Build history of the part. All positions in model axes, mm. Face numbers are marked on the shaded views. A direction names the side the tool comes from. Coordinates: 2 decimals unless noted, no trailing zeros.
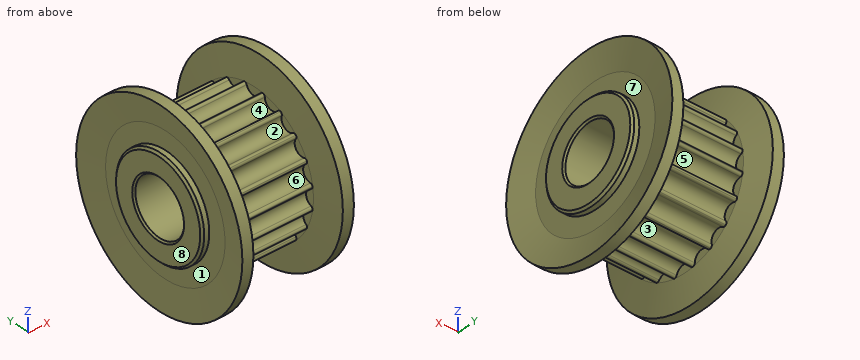
```python
from build123d import *

# Parameters (mm, degrees)
CUT_EXTRUDE_START        = 1.65
CUT_EXTRUDE_1_DEPTH      = 7
PATTERN_CIRCULAR_1_COUNT = 20
SKETCH_6_R               = 2.5
CUT_EXTRUDE_2_DEPTH      = 11.3
CHAMFER_1_SIZE           = 0.15


with BuildPart() as part:
    # Sketch 3 → Revolve 1 (revolve)
    with BuildSketch(Plane.XY):
        Polygon((0, 0), (0, 4.31), (0.19, 4.5), (1.65, 4.5), (1.65, 6.11), (8.65, 6.11), (8.65, 4.5), (10.11, 4.5), (10.3, 4.31), (10.3, 0), align=None)
    revolve(axis=Axis((10.3, 0, 0), (-1, 0, 0)))

    # Sketch 4 → Cut-Extrude 1 (cut)
    with BuildSketch(Plane(origin=(0, 0, 0), x_dir=(0, 0, -1), z_dir=(1, 0, 0)).offset(CUT_EXTRUDE_START)):
        with BuildLine():
            ThreePointArc((0.968009552, 6.032831633), (0.81174441, 6.002056879), (0.712936658, 5.877145279))
            ThreePointArc((0.712936658, 5.877145279), (0, 5.36), (-0.712936658, 5.877145279))
            ThreePointArc((-0.712936658, 5.877145279), (-0.81174441, 6.002056879), (-0.968009552, 6.032831633))
            ThreePointArc((-0.968009552, 6.032831633), (0, 6.11), (0.968009552, 6.032831633))
        make_face()
    cut_extrude_1 = extrude(amount=CUT_EXTRUDE_1_DEPTH, mode=Mode.SUBTRACT)

    # Pattern Circular 1: Cut-Extrude 1 ×20 about axis
    pattern_circular_1_axis = Axis((0, 0, 0), (1, 0, 0))
    for i in range(1, PATTERN_CIRCULAR_1_COUNT):
        add(cut_extrude_1.rotate(pattern_circular_1_axis, i * 360 / PATTERN_CIRCULAR_1_COUNT), mode=Mode.SUBTRACT)

    # Sketch 5 → Revolve 2 (revolve)
    with BuildSketch(Plane.XY):
        Polygon((1.1, 8.5), (1.65, 6.11), (1.65, 4.5), (0.65, 4.5), (0.65, 6.11), (0.1, 8.5), align=None)
        Polygon((9.65, 4.5), (8.65, 4.5), (8.65, 6.11), (9.2, 8.5), (10.2, 8.5), (9.65, 6.11), align=None)
    revolve(axis=Axis((0, 0, 0), (1, 0, 0)))

    # Sketch 6 → Cut-Extrude 2 (cut, through all)
    with BuildSketch(Plane(origin=(0, 0, 0), x_dir=(0, 0, -1), z_dir=(1, 0, 0))):
        Circle(SKETCH_6_R)
    extrude(amount=CUT_EXTRUDE_2_DEPTH, mode=Mode.SUBTRACT)

    # Chamfer 1
    chamfer_1_edges = [part.edges().sort_by_distance(p)[0] for p in [
        (0, 0, 2.5),
        (10.3, 0, 2.5),
    ]]
    chamfer(chamfer_1_edges, length=CHAMFER_1_SIZE)


solid = part.part
```
1. 3-axis set-ups, long thin cutter, end or side, ignore diameter. For the marked faces 1, 2, 3, 4 and 5: which of +Z, -Z, +X, -X, +Y, -Y reach the whole face in a straight line?
Computed values:
face 1: -X
face 2: none
face 3: -Z
face 4: +Z
face 5: +Y
2. Flat gauge pins, fed straight in: pin 1 (5 mm diameter, centred on y = 5, z = 5.5, fed in from +X); pin 2 (1.5 mm diameter, centred on y = -4.5, z = 4, fed in from -X); pin 3 (5 mm diameter, centred on x = 2, y = -2.5, fed in from -Z). Where does each tip first touch, or does it go through?
Computed values:
pin 1: stops at x = 10.2
pin 2: stops at x = 0.5
pin 3: stops at z = -8.5
3. Mould opens along X. For the marked faces 6, 7 and 8 say: +X half, -X half, draft (parallel to the pull), parting line (faces both ways), or undercut.
Computed values:
face 6: undercut
face 7: +X half
face 8: -X half
4. Probe line 1 along X through (y, z) = (5.25, -2.25); line 2 along X through (y, z) = (-4.75, 0.75); line 3 along Z through (x, y) = (1, -1). List the from-to ranges inside material, lowest first.
Computed values:
line 1: x = 0.65 to 1.65, 8.65 to 9.65
line 2: x = 0.65 to 9.65
line 3: z = -8.44 to -2.29, 2.29 to 8.44
